Geometry: final body of the model. Coordinates: model frame, mm. A direction names the side the tool comes from. Give positions to 0.01 mm unless a question says otherwise; leave off trailing zeros. Order: outer loops, then holes, each group sorted by start corner. A loop starts at its lowest first (then second) coordinate and runs counter-clockwise, first axis right, second up. Notation, with made-up numbers: (80, -11.75) -> (87, -11.75) arc R19 ccw to (87, 12.25) -> close; hole circle Ø1 at (38.5, 28). An arc over 180 degrees is marked (long way). One line per question, with ' | ' between items. Start each with the question number.
(1) Mould query, pull axis Y, two halves, no side actions, for faces 1 (the face through (0.24, -15.44, -2.97)), 2 (the face through (1.99, 6.13, 2.46)), 3 (the face through (-12.5, 0, -3)). Classes: +Y half, -Y half, draft (parallel to the pull), parting line (faces both ways), or undercut.
(2) Section B-B (x = -15). Return loops of the section in (y, z), then the cut area to 3 significant figures.
(3) Section C-C (x = -4.5). State how many separate pieces and enclosed holes the cut face has, then the cut area to 3 significant figures.
(4) Set-up query: faces 4 (the face through (14.755, -4.54, -2.969)), 5 (the face through (10.154, 7.291, -2.535)), 6 (the face through (-15, -5, -3)). Return all of +Z, -Z, +X, -X, +Y, -Y with unobstructed straight access to the full face (end or side cutting, diameter ignored); none if empty.
(5) Ray query, L1, parallel to Y at x = -0.5, z = 1.5; L2, parallel to X at y = 3.5, z = -5.5; L3, parallel to Z at x = 6, y = -14. Return the intervals inside material, ascending.
(6) First-contact query: pin 1 Ø4.5 at (x, z) = (-13.5, -4.5) entering from +Y; pin 2 Ø4.5 at (x, y) = (-1.61, -7.84) entering from -Z; pin 3 Ø4 at (y, z) = (0.5, -2.5) entering from +X; pin 4 Ø4 at (x, z) = (5, -5) entering from +Y. Flat tips, straight axial feed; report the tip coordinate or a pass-through.
(7) Section A-A (z = -1.25). Return loops of the section in (x, y).
(8) Section D-D (z = 2.75). Return loops of the section in (x, y) (3 decimals), then the cut area to 3 significant figures.
```python
from build123d import *
from build123d.topology import SkipClean

# Parameters (mm, degrees)
ESQUISSE1_R                  = 17.5
ESQUISSE1_R_2                = 5.125
BOSS_EXTRU_1_DEPTH           = 5
ESQUISSE2_R                  = 1.5
BOSS_EXTRU_2_DEPTH           = 5
ENL_V_MAT_EXTRU_1_DEPTH      = 26.860201082
R_P_TITION_CIRCULAIRE1_COUNT = 5
ESQUISSE4_R                  = 1.75
ENL_V_MAT_EXTRU_2_DEPTH      = 10


with BuildPart() as part:
    # Esquisse1 → Boss.-Extru.1 (new body)
    with BuildSketch(Plane.XY):
        Circle(ESQUISSE1_R)
        Circle(ESQUISSE1_R_2, mode=Mode.SUBTRACT)
    extrude(amount=BOSS_EXTRU_1_DEPTH)

    # Esquisse2 → Boss.-Extru.2 (add, symmetric)
    with BuildSketch(Plane(origin=(0, 0, 0), x_dir=(1, 0, 0), z_dir=(0, 1, 0))):
        with BuildLine():
            Line((-17.5, 0), (-17.5, 5))
            ThreePointArc((-17.5, 5), (-15, 7.5), (-12.5, 5))
            Line((-12.5, 5), (-12.5, 0))
            Line((-12.5, 0), (-17.5, 0))
        make_face()
        with Locations(Location((-15, 5, 0), (0, 0, 270))):
            Circle(ESQUISSE2_R, mode=Mode.SUBTRACT)
    boss_extru_2 = extrude(amount=BOSS_EXTRU_2_DEPTH, both=True)

    # Esquisse3 → Enl_v. mat.-Extru.1 (cut, through all)
    with SkipClean():  # the faces are left unmerged after this step: merging them gives an invalid solid
        with BuildSketch(Plane.XY):
            with BuildLine():
                ThreePointArc((-16.770509831, -5), (-17.316667145, -2.526467688), (-17.5, 0))
                Line((-17.5, 0), (-17.5, -5))
                Line((-17.5, -5), (-16.770509831, -5))
            make_face()
            with BuildLine():
                Line((-17.5, 5), (-17.5, 0))
                ThreePointArc((-17.5, 0), (-17.316667145, 2.526467688), (-16.770509831, 5))
                Line((-16.770509831, 5), (-17.5, 5))
            make_face()
        enl_v_mat_extru_1 = extrude(amount=-ENL_V_MAT_EXTRU_1_DEPTH, mode=Mode.SUBTRACT)

    # R_p_tition circulaire1: Boss.-Extru.2, Enl_v. mat.-Extru.1 ×5 about axis
    with SkipClean():  # the faces are left unmerged after this step: merging them gives an invalid solid
        r_p_tition_circulaire1_axis = Axis((0, 0, 0), (0, 0, 1))
        add([boss_extru_2.rotate(r_p_tition_circulaire1_axis, i * 360 / R_P_TITION_CIRCULAIRE1_COUNT) for i in range(1, R_P_TITION_CIRCULAIRE1_COUNT)])
        add([enl_v_mat_extru_1.rotate(r_p_tition_circulaire1_axis, i * 360 / R_P_TITION_CIRCULAIRE1_COUNT) for i in range(1, R_P_TITION_CIRCULAIRE1_COUNT)], mode=Mode.SUBTRACT)

    # Esquisse4 → Enl_v. mat.-Extru.2 (cut)
    with SkipClean():  # the faces are left unmerged after this step: merging them gives an invalid solid
        with BuildSketch(Plane(origin=(0, 0, 0), x_dir=(-1, 0, 0), z_dir=(0, 0, -1))):
            with Locations((-7.836351046, -1.609845421)):
                Circle(ESQUISSE4_R)
            with Locations((1.609845421, -7.836351046)):
                Circle(ESQUISSE4_R)
            with Locations((7.836351046, 1.609845421)):
                Circle(ESQUISSE4_R)
            with Locations((-1.609845421, 7.836351046)):
                Circle(ESQUISSE4_R)
        extrude(amount=-ENL_V_MAT_EXTRU_2_DEPTH, mode=Mode.SUBTRACT)


solid = part.part
```
Response:
1) face 1: -Y half | face 2: undercut | face 3: draft
2) outline: (-9.01, 0) -> (-5, 0) -> (-5, -3.5) -> (5, -3.5) -> (5, 0) -> (9.01, 0) -> (9.01, 5) -> (-9.01, 5) -> close; (-5, -7.5) -> (5, -7.5) -> (5, -6.5) -> (-5, -6.5) -> close | area: 135 mm^2
3) separate pieces: 2 | enclosed holes: 2 | area: 203 mm^2
4) face 4: -Z, +X | face 5: -Z | face 6: -Z, -X, -Y
5) L1: y = -17.49 to -9.19, -6.48 to -5.1, 5.1 to 17.49 | L2: x = -17.15 to -16.41, -13.59 to -12.55, 12.97 to 13.32 | L3: z = 0 to 5
6) pin 1: stops at y = 5 | pin 2: stops at z = 0 | pin 3: stops at x = -12.5 | pin 4: passes through
7) outline: (-16.77, -5) -> (-12.5, -5) -> (-12.5, 5) -> (-16.77, 5) arc R17.5 ccw to start; (-9.94, -14.4) arc R17.5 ccw to (-0.43, -17.49) -> (0.89, -13.43) -> (-8.62, -10.34) -> close; (-9.94, 14.4) -> (-8.62, 10.34) -> (0.89, 13.43) -> (-0.43, 17.49) arc R17.5 ccw to start; (7.17, -11.39) -> (10.63, -13.9) arc R17.5 ccw to (16.51, -5.81) -> (13.05, -3.3) -> close; (7.17, 11.39) -> (13.05, 3.3) -> (16.51, 5.81) arc R17.5 ccw to (10.63, 13.9) -> close
8) outline: circle Ø35 at (0, 0); hole circle Ø3.5 at (-7.836, 1.61); hole circle Ø10.25 at (0, 0); hole circle Ø3.5 at (-1.61, -7.836); hole circle Ø3.5 at (1.61, 7.836); hole circle Ø3.5 at (7.836, -1.61) | area: 841 mm^2
